Source: CAD feature listing. Evaluate the final solid. Frame: model axes, mm. A direction names the side the tool comes from. Round coordinates to 2 decimals unless told otherwise and drop trailing zeros. Loops run counter-clockwise (first coordinate to the right, second up) from the corner with the lowest first, then second, coordinate; pieces in that order, holes last. Notation, with made-up numbers: M -8.75,7 L 16.25,7 A23 ccw 16.25,34 Z; hole C 17.5,29 d10. An arc over 180 degrees is marked long. Answer as a JSON object with one key per item and string values.
from build123d import *

# Parameters (mm, degrees)
SKETCH1_W           = 35
SKETCH1_H           = 28.5
BOSS_EXTRUDE1_DEPTH = 25
SKETCH2_R           = 4.25
CUT_EXTRUDE1_DEPTH  = 20
SKETCH3_R           = 11.25
CUT_EXTRUDE2_DEPTH  = 7.5
SKETCH9_W           = 35
SKETCH9_H           = 5
BOSS_EXTRUDE4_DEPTH = 22
SKETCH4_W           = 4
SKETCH4_H           = 47
BOSS_EXTRUDE2_DEPTH = 20
FILLET1_R           = 1.5
CUT_EXTRUDE3_REACH  = 66.415
SKETCH6_R           = 2.15
MIRROR1_START       = -14.2
MIRROR1_OUTLINE_W   = 20
MIRROR1_OUTLINE_H   = 47
MIRROR1_OUTLINE_R   = 2.15
MIRROR1_DEPTH       = 4
MIRROR1_2_DEPTH     = 47
FILLET2_R           = 1.5


with BuildPart() as part:
    # Sketch1 → Boss-Extrude1 (new body)
    with BuildSketch(Plane.XY):
        with BuildLine():
            ThreePointArc((-17.5, 14.25), (0, 31.75), (17.5, 14.25))
            Line((17.5, 14.25), (-17.5, 14.25))
        make_face()
        Rectangle(SKETCH1_W, SKETCH1_H)
    extrude(amount=BOSS_EXTRUDE1_DEPTH)

    # Sketch2 → Cut-Extrude1 (cut)
    with BuildSketch(Plane.XY.offset(25)):
        with Locations((0, 9.25)):
            Circle(SKETCH2_R)
    extrude(amount=-CUT_EXTRUDE1_DEPTH, mode=Mode.SUBTRACT)

    # Sketch3 → Cut-Extrude2 (cut)
    with BuildSketch(Plane.XY.offset(25)):
        with Locations((0, 9.25)):
            Circle(SKETCH3_R)
    extrude(amount=-CUT_EXTRUDE2_DEPTH, mode=Mode.SUBTRACT)

    # Sketch9 → Boss-Extrude4 (add)
    with BuildSketch(Plane.XY.offset(25)):
        with Locations((0, -11.75)):
            Rectangle(SKETCH9_W, SKETCH9_H)
    extrude(amount=BOSS_EXTRUDE4_DEPTH)

    # Sketch4 → Boss-Extrude2 (add)
    with BuildSketch(Plane.XZ.offset(14.25)):
        with Locations((12.2, 23.5)):
            Rectangle(SKETCH4_W, SKETCH4_H)
    extrude(amount=BOSS_EXTRUDE2_DEPTH)

    # Fillet1
    fillet1_edges = [part.edges().sort_by_distance(p)[0] for p in [
        (14.2, -14.25, 23.5),
        (17.5, -14.25, 23.5),
    ]]
    fillet(fillet1_edges, radius=FILLET1_R)

    # Sketch6 → Cut-Extrude3 (cut, up to next)
    with BuildSketch(Plane.ZY.offset(-10.2), mode=Mode.PRIVATE) as cut_extrude3_sk1:
        with Locations(Location((6, -24.25, 0), (0, 0, 270))):
            Circle(SKETCH6_R)
    cut_extrude3_tool1 = extrude(cut_extrude3_sk1.sketch, amount=-CUT_EXTRUDE3_REACH, mode=Mode.PRIVATE) & part.part
    # Sketch6 → Cut-Extrude3 (cut, up to next)
    with BuildSketch(Plane.ZY.offset(-10.2), mode=Mode.PRIVATE) as cut_extrude3_sk2:
        with Locations(Location((41, -24.25, 0), (0, 0, 270))):
            Circle(SKETCH6_R)
    cut_extrude3_tool2 = extrude(cut_extrude3_sk2.sketch, amount=-CUT_EXTRUDE3_REACH, mode=Mode.PRIVATE) & part.part
    add(cut_extrude3_tool1.solids().sort_by_distance((10.2, -24.25, 6))[0], mode=Mode.SUBTRACT)
    add(cut_extrude3_tool2.solids().sort_by_distance((10.2, -24.25, 41))[0], mode=Mode.SUBTRACT)

    # Mirror1: read off the stored shape, not the designer's step
    # Mirror1 outline → Mirror1 (add)
    with BuildSketch(Plane.YZ.offset(MIRROR1_START)):
        with Locations((-24.25, 23.5)):
            Rectangle(MIRROR1_OUTLINE_W, MIRROR1_OUTLINE_H)
        with Locations((-24.25, 6)):
            Circle(MIRROR1_OUTLINE_R, mode=Mode.SUBTRACT)
        with Locations((-24.25, 41)):
            Circle(MIRROR1_OUTLINE_R, mode=Mode.SUBTRACT)
    extrude(amount=MIRROR1_DEPTH)

    # Mirror1 2 outline → Mirror1 2 (add)
    with BuildSketch(Plane.XY):
        with BuildLine():
            Line((-14.2, -14.25), (-15.7, -14.25))
            ThreePointArc((-15.7, -14.25), (-14.639339828, -14.689339828), (-14.2, -15.75))
            Line((-14.2, -15.75), (-14.2, -14.25))
        make_face()
    extrude(amount=MIRROR1_2_DEPTH)

    # Fillet2
    fillet2_edges = [part.edges().sort_by_distance(p)[0] for p in [
        (-17.5, 2.5, 25),
        (17.5, 2.5, 25),
        (-17.5, -9.25, 36),
        (0, -9.25, 25),
        (17.5, -9.25, 36),
        (-16.6, -14.25, 47),
        (0, -9.25, 47),
        (14.2, -25, 47),
        (14.2, -34.25, 23.5),
        (0, 31.75, 25),
        (17.5, -11, 47),
        (15.85, -14.25, 47),
        (17.060660172, -13.810660172, 47),
        (14.639339828, -14.689339828, 47),
        (-14.2, -34.25, 23.5),
        (-14.2, -25, 47),
        (-14.639339828, -14.689339828, 47),
        (-17.5, -14.25, 23.5),
    ]]
    fillet(fillet2_edges, radius=FILLET2_R)


solid = part.part
Item 1: Contact query for flat-ended pins moving along their axis: pin 1 Ø13.5 at (y, z) = (-20.5, 26.5) entering from -X; pin 2 Ø1.5 at (x, z) = (3.5, 25) entering from +Y; pin 3 Ø7 at (x, y) = (-5.5, 14.5) entering from +Z. Output: stop coordinate, or through.
Answer sheet:
{"pin 1": "stops at x = -17.12", "pin 2": "stops at y = 31.22", "pin 3": "stops at z = 17.5"}
Item 2: Access query for faces 4 (the cylindrical face through (-17.07, 3.4, 24.55)), 5 (the flat face through (10.2, -24, 23)), 6 (the flat face through (5, 9, 17.5)). Directions: +Z, -Z, +X, -X, +Y, -Y. A direction counts if a zero-diameter tool reaches every point of the face in a straight line with its end or side. Return the directions, or none.
Answer sheet:
{"face 4": "+Z, -X, +Y", "face 5": "+Z, -Z, -Y", "face 6": "+Z"}
Item 3: Section D-D on y = 2.5. Return the cut outline in (x, z), then the cut area to 3 significant figures.
Answer sheet:
{"outline": "M -17.5,0 L 17.5,0 L 17.5,23.5 A1.5 ccw 16,25 L 9,25 L 9,17.5 L -9,17.5 L -9,25 L -16,25 A1.5 ccw -17.5,23.5 Z", "area": "739 mm²"}
Item 4: Pull-direction query (Y, two-part tool) for faces 1 (the cylindrical face through (12.17, -26.3, 6.65)), 2 (the flat face through (14.2, -24, 22)), 3 (the cylindrical face through (0.22, -8.82, 25.45)); classes: pulls with the +Y half, pulls with the -Y half, needs draft (parallel to the pull), parting line crosses it, or undercut.
Answer sheet:
{"face 1": "undercut", "face 2": "needs draft", "face 3": "pulls with the +Y half"}
Item 5: Section C-C on z = 41. Return the cut outline in (x, y), then the cut area to 3 significant figures.
Answer sheet:
{"outline": "M -17.5,-12.75 A1.5 ccw -16,-14.25 L -15.7,-14.25 A1.5 cw -14.2,-15.75 L -14.2,-22.1 L -10.2,-22.1 L -10.2,-14.25 L 10.2,-14.25 L 10.2,-22.1 L 14.2,-22.1 L 14.2,-15.75 A1.5 cw 15.7,-14.25 L 16,-14.25 A1.5 ccw 17.5,-12.75 L 17.5,-10.75 A1.5 ccw 16,-9.25 L -16,-9.25 A1.5 ccw -17.5,-10.75 Z; M -14.2,-32.75 A1.5 ccw -12.7,-34.25 L -10.2,-34.25 L -10.2,-26.4 L -14.2,-26.4 Z; M 10.2,-34.25 L 12.7,-34.25 A1.5 ccw 14.2,-32.75 L 14.2,-26.4 L 10.2,-26.4 Z", "area": "299 mm²"}
Item 6: Line query: probe 1 along Z at (x, y) = (12.3, -24.25); probe 2 along X at (y, z) = (-21, 4.5); probe 3 along Y at (x, z) = (0, 21). Output: solid intervals per line, ascending. Write a range as from..to.
Answer sheet:
{"probe 1": "z = 0..3.85, 8.15..38.85, 43.15..47", "probe 2": "x = -14.2..-10.2, 10.2..14.2", "probe 3": "y = -14.25..-2, 20.5..31.75"}
Item 7: Section B-B on y = -24.25. Return the cut outline in (x, z).
Answer sheet:
{"outline": "M -14.2,0 L -10.2,0 L -10.2,3.85 L -14.2,3.85 Z; M -14.2,8.15 L -10.2,8.15 L -10.2,38.85 L -14.2,38.85 Z; M -14.2,43.15 L -10.2,43.15 L -10.2,47 L -12.7,47 A1.5 ccw -14.2,45.5 Z; M 10.2,0 L 14.2,0 L 14.2,3.85 L 10.2,3.85 Z; M 10.2,8.15 L 14.2,8.15 L 14.2,38.85 L 10.2,38.85 Z; M 10.2,43.15 L 14.2,43.15 L 14.2,45.5 A1.5 ccw 12.7,47 L 10.2,47 Z"}
Item 8: Section A-A on z = 6. Return the cut outline in (x, y), then the cut area to 3 significant figures.
Answer sheet:
{"outline": "M -17.5,-12.75 A1.5 ccw -16,-14.25 L -15.7,-14.25 A1.5 cw -14.2,-15.75 L -14.2,-22.1 L -10.2,-22.1 L -10.2,-14.25 L 10.2,-14.25 L 10.2,-22.1 L 14.2,-22.1 L 14.2,-15.75 A1.5 cw 15.7,-14.25 L 16,-14.25 A1.5 ccw 17.5,-12.75 L 17.5,14.25 A17.5 ccw -17.5,14.25 Z; M -14.2,-32.75 A1.5 ccw -12.7,-34.25 L -10.2,-34.25 L -10.2,-26.4 L -14.2,-26.4 Z; M 10.2,-34.25 L 12.7,-34.25 A1.5 ccw 14.2,-32.75 L 14.2,-26.4 L 10.2,-26.4 Z; hole C 0,9.25 d8.5", "area": "1,550 mm²"}
